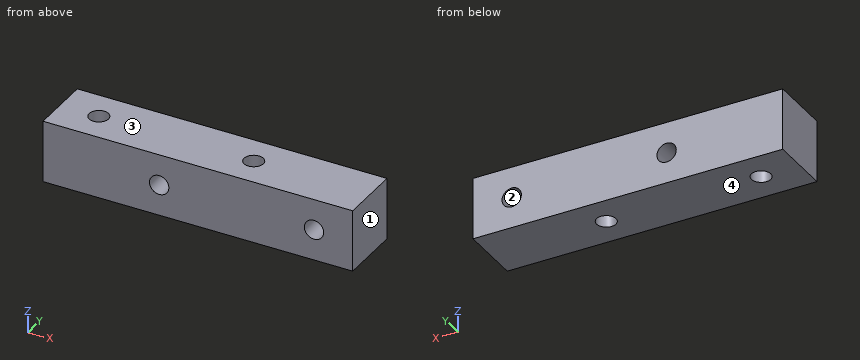
```python
from build123d import *

# Parameters (mm, degrees)
SKETCH_1_W                   = 40
SKETCH_1_H                   = 8
EXTRUDE_1_DEPTH              = 8
HOLE_WIZARD_M3_1_D           = 2.5
HOLE_WIZARD_M3_1_ON_FACE_2_D = 2.5


with BuildPart() as part:
    # 草图1 → 凸台-拉伸1 (new body)
    with BuildSketch(Plane.XY):
        Rectangle(SKETCH_1_W, SKETCH_1_H)
    extrude(amount=EXTRUDE_1_DEPTH)

    # M3 螺纹孔的螺纹孔钻头1 (through all)
    with Locations(Plane(origin=(-5, 4, 4), x_dir=(1, 0, 0), z_dir=(0, 1, 0))):
        with Locations((0, 0), (20, 0)):
            Hole(HOLE_WIZARD_M3_1_D / 2)

    # M3 螺纹孔的螺纹孔钻头1 on face 2 (through all)
    with Locations(Plane(origin=(5, 0, 8), x_dir=(1, 0, 0), z_dir=(0, 0, 1))):
        with Locations((0, 0), (-20, 0)):
            Hole(HOLE_WIZARD_M3_1_ON_FACE_2_D / 2)


solid = part.part
```
Geometry: final body of the model. Coordinates: model frame, mm. Face numbers are marked on the shaded views. Give positions to 0.01 mm unless a question says otherwise; leave off trailing zeros. Loops run counter-clockwise (first coordinate to the right, second up) from the corner with the lowest first, then second, coordinate; pieces in that order, holes last. Notation, with made-up numbers: (42, 29.25) -> (87, 29.25) arc R21 ccw to (87, 40.25) -> close; hole circle Ø4 at (36.5, 46.5). An arc over 180 degrees is marked (long way). Use one line per item in the form item = value.
Item 1: Section query C-C on x = -5. Output: boundary loops of the cut face in (y, z).
A:
outline = (-4, 0) -> (4, 0) -> (4, 2.75) -> (-4, 2.75) -> close; (-4, 5.25) -> (4, 5.25) -> (4, 8) -> (-4, 8) -> close
Item 2: Line query: probe 1 along X at (y, z) = (-2.75, 4); probe 2 along Z at (x, y) = (15, 0.25); probe 3 along X at (y, z) = (-0.25, 4). Output: solid intervals per line, ascending.
A:
probe_1 = -20 to -6.25, -3.75 to 13.75, 16.25 to 20
probe_2 = 0 to 2.75, 5.25 to 8
probe_3 = -20 to -16.22, -13.78 to -6.25, -3.75 to 3.78, 6.22 to 13.75, 16.25 to 20
Item 3: Section query A-A on y = 0. Output: boundary loops of the cut face in (x, z), and give its area (3 significant figures).
A:
outline = (-20, 0) -> (-16.25, 0) -> (-16.25, 8) -> (-20, 8) -> close; (-13.75, 0) -> (3.75, 0) -> (3.75, 8) -> (-13.75, 8) -> close; (6.25, 0) -> (20, 0) -> (20, 8) -> (6.25, 8) -> close; hole circle Ø2.5 at (-5, 4); hole circle Ø2.5 at (15, 4)
area = 270 mm^2
Item 4: Section query D-D on z = 1.25. Output: boundary loops of the cut face in (x, y), and give its area (3 significant figures).
A:
outline = (-20, -4) -> (20, -4) -> (20, 4) -> (-20, 4) -> close; hole circle Ø2.5 at (-15, 0); hole circle Ø2.5 at (5, 0)
area = 310 mm^2
Item 5: Section query B-B on z = 4.75. Output: boundary loops of the cut face in (x, y).
A:
outline = (-20, -4) -> (-6, -4) -> (-6, 4) -> (-20, 4) -> close; (-4, -4) -> (14, -4) -> (14, 4) -> (-4, 4) -> close; (16, -4) -> (20, -4) -> (20, 4) -> (16, 4) -> close; hole circle Ø2.5 at (-15, 0); hole circle Ø2.5 at (5, 0)
Item 6: Draft query along Z for the marked faces 1, 2, 3 and 4. Return one class per face: pulls with the +Z half, pulls with the -Z half, needs draft (parallel to the pull), parting line crosses it, or undercut.
A:
face_1 = needs draft
face_2 = undercut
face_3 = pulls with the +Z half
face_4 = pulls with the -Z half
